Study the drawing (mm; zero at the part's minimum x, y, z) and answer. A direction names the side the tool comes from. Round coordinates to 2 decimals unless told otherwise and drop trailing zeros. Write each loop counter-clockwise with the first axis right and the second up, starting at its lowest first coordinate (ties: lowest second). Pieces come first, ordered by that corner, then holes.
(1) A cutting plane is placed at C-C, the plane z = 19. Give the vertices of the cut face in (x, y), and give its area (3 significant figures).
(2) For the marked faces 1, 2, 3 and 4, determine the directions among +Z, -Z, +X, -X, +Y, -Y from which every point of the face is accessible in a straight line to the end or side of a thin tool.
(3) Find the intervals of material crossed by probe 1 along X at (y, z) = (33.6, 12); probe 2 along Y at (x, z) = (24.5, 3.75); probe 3 along X at (y, z) = (28.5, 7.5), in increasing order.
(4) A cutting plane is placed at D-D, the plane y = 17. Give the vertices of the cut face in (x, z).
(5) A cutting plane is placed at A-A, the plane y = 25. Give the vertices of the cut face in (x, z), and give its area (3 significant figures).
(6) A cutting plane is placed at B-B, the plane x = 22. Give the vertices of the cut face in (y, z), and give its area (3 significant figures).
(7) Each of these flat-tipped pins is pushed along its axis until it touches: pin 1 Ø3 at (x, z) = (165.5, 9) entering from +Y; pin 2 Ø8 at (x, y) = (170, 10) entering from +Z; pin 3 Ø10 at (x, y) = (93.5, 16.5) entering from +Z. Where does it stop, or does it pass through?
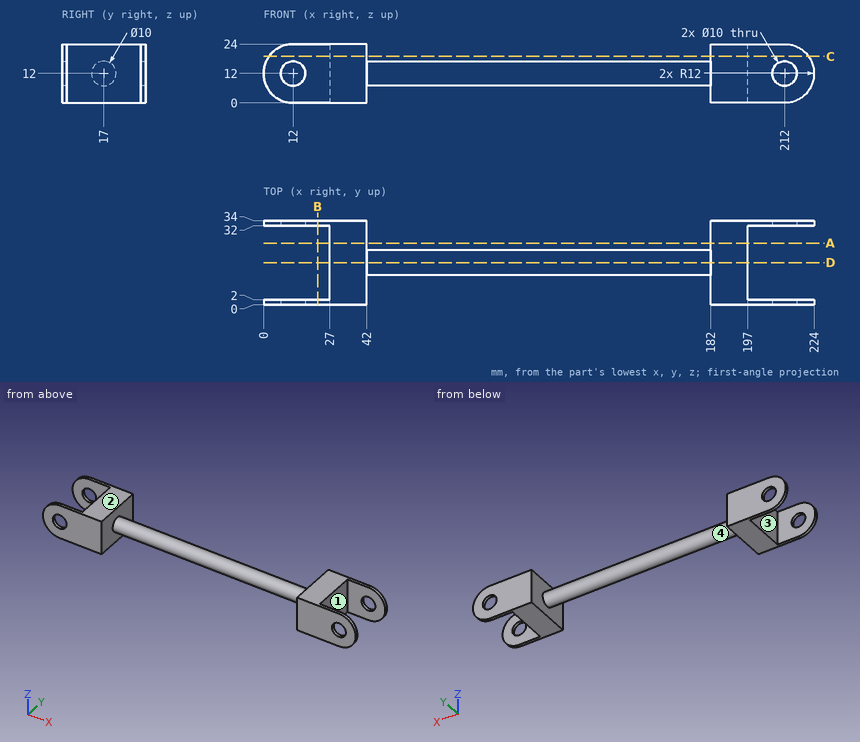
Solutions:
1. outline: (2.25, 0) - (42, 0) - (42, 34) - (2.25, 34) - (2.25, 32) - (27, 32) - (27, 2) - (2.25, 2) - close; (182, 0) - (221.75, 0) - (221.75, 2) - (197, 2) - (197, 32) - (221.75, 32) - (221.75, 34) - (182, 34) - close
1. area: 1,220 mm2
2. face 1: +Z, -Z, +X
2. face 2: +Z, +X, -X, +Y, -Y
2. face 3: +Z, -Z, -X
2. face 4: none
3. probe 1: x = 0 to 7, 17 to 42, 182 to 207, 217 to 224
3. probe 2: y = 0 to 2, 32 to 34
3. probe 3: x = 27 to 42, 182 to 197
4. outline: (27, 0) - (42, 0) - (42, 7) - (182, 7) - (182, 0) - (197, 0) - (197, 24) - (182, 24) - (182, 17) - (42, 17) - (42, 24) - (27, 24) - close
5. outline: (27, 0) - (42, 0) - (42, 24) - (27, 24) - close; (182, 0) - (197, 0) - (197, 24) - (182, 24) - close
5. area: 720 mm2
6. outline: (0, 0) - (2, 0) - (2, 24) - (0, 24) - close; (32, 0) - (34, 0) - (34, 24) - (32, 24) - close
6. area: 96.0 mm2
7. pin 1: stops at y = 21.77
7. pin 2: stops at z = 16
7. pin 3: stops at z = 17
